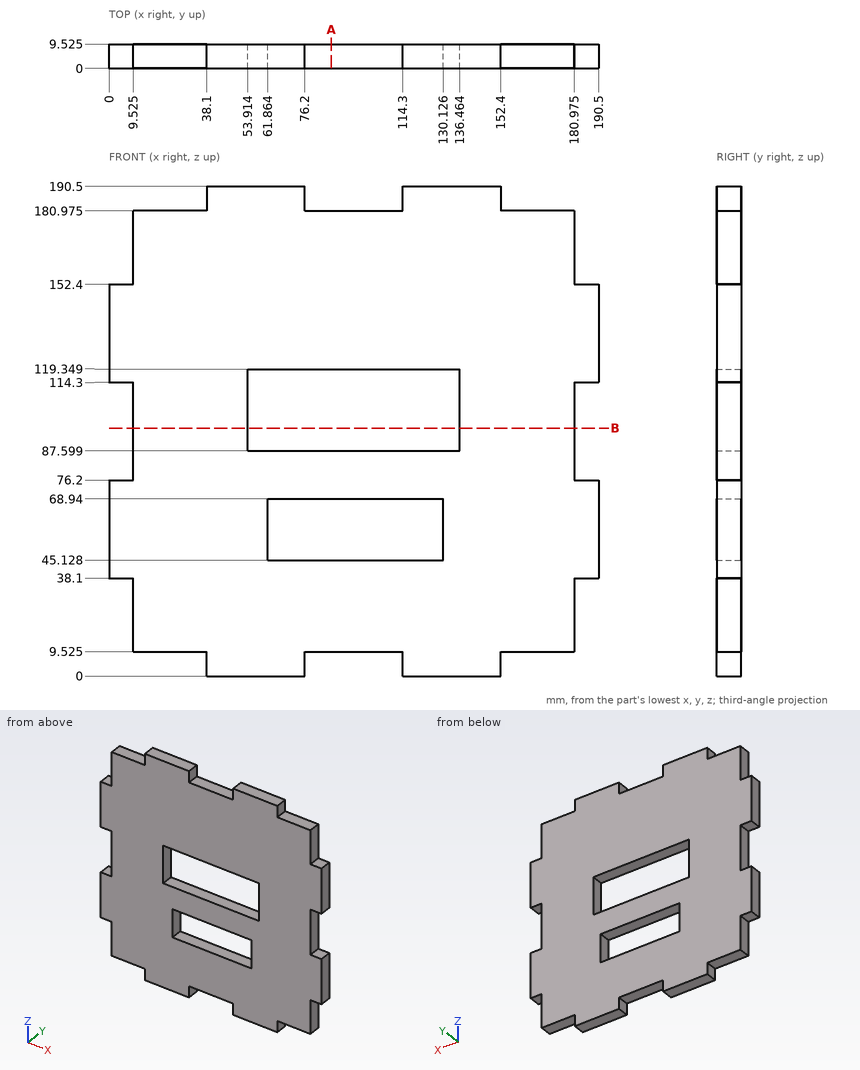
Geometry: see drawing. Coordinates: mm, zero at the bounding-box minimum. Coordinates: 2 decimals unless noted, no trailing zeros. Order: outer loops, then holes, each group sorted by start corner. A loop starts at its lowest first (then second) coordinate and runs counter-clockwise, first axis right, second up. Notation, with made-up numbers: M -15,-35 L 3,-35 A25 ccw 3,-12 Z; hole C 61.25,54 d5. An arc over 180 degrees is marked long. Answer in a Markdown table with one row per item. Add a question column.
Q1. Section query B-B on z = 96.5. Return the cut outline in (x, y) (1 decimal).
Q2. Section query A-A on x = 86.5. Count the separate pieces of the cut face and the enclosed holes in it, and give its area (3 significant figures).
Q3. Contact query for flat-ended pins moving along their axis: P1, Ø3, axis at y = 3.5, z = 187, coming from the -X side; P2, Ø3, axis at y = 5, z = 99.5, coming from the -X side (1 decimal); P3, Ø5, axis at x = 23.5, y = 2.5, coming from the +Z side (1 decimal). Output: stop coordinate, or through.
Q4. Line query: L1, parallel to X at y = 7, z = 54; L2, parallel to Z at x = 118, y = 6.25; L3, parallel to X at y = 8.25, z = 96.5 (1 decimal). Output: solid intervals per line, ascending.
Completed:
| question | item | result |
|---|---|---|
| 1 | outline | M 9.5,0 L 53.9,0 L 53.9,9.5 L 9.5,9.5 Z; M 136.5,0 L 181,0 L 181,9.5 L 136.5,9.5 Z |
| 2 | separate pieces | 3 |
| 2 | enclosed holes | 0 |
| 2 | area | 1,100 mm2 |
| 3 | P1 | stops at x = 38.1 |
| 3 | P2 | stops at x = 9.5 |
| 3 | P3 | stops at z = 181 |
| 4 | L1 | x = 0 to 61.86, 130.13 to 190.5 |
| 4 | L2 | z = 0 to 45.13, 68.94 to 87.6, 119.35 to 190.5 |
| 4 | L3 | x = 9.5 to 53.9, 136.5 to 181 |
